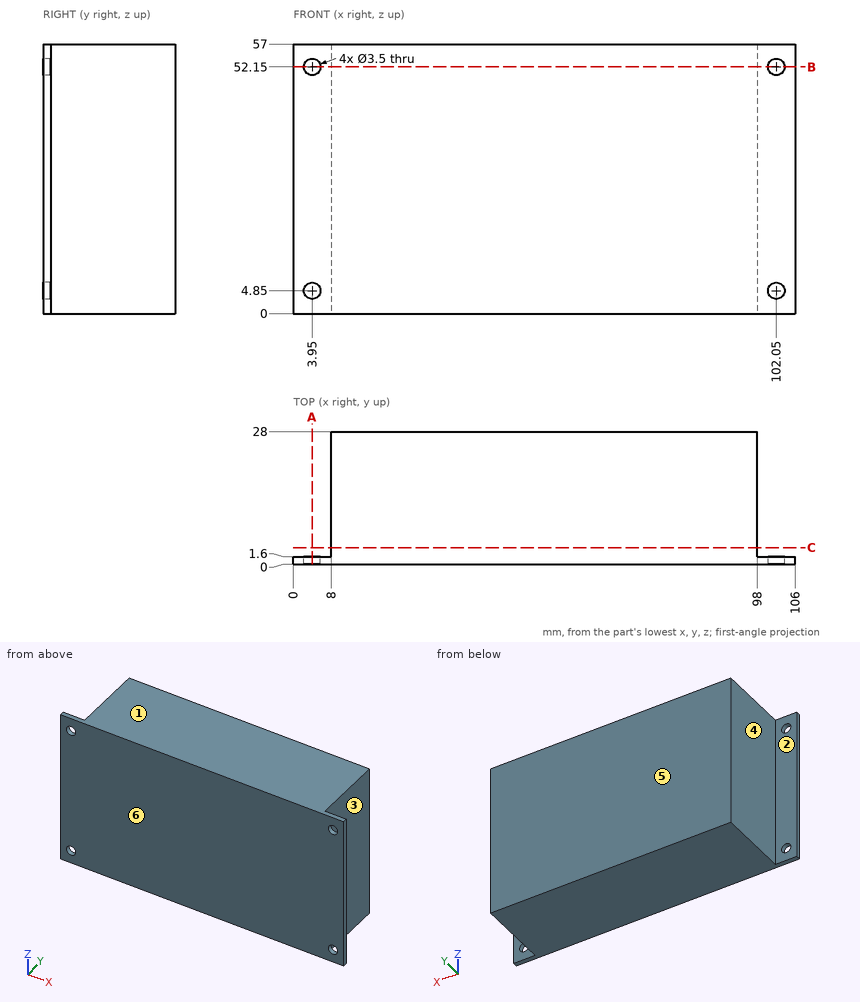
Source: three-view drawing plus pictorial views. Frame: mm from the lowest corner of the part. A direction names the side the tool comes from. Give positions to 0.01 mm unless a question says otherwise; leave off trailing zeros. Loops run counter-clockwise (first coordinate to the right, second up) from the corner with the lowest first, then second, coordinate; pieces in that order, holes last. Notation, with made-up numbers: (-24, 65.5) -> (31, 65.5) arc R22 cw to (31, 71.5) -> close; hole circle Ø5 at (25.25, 83). An arc over 180 degrees is marked (long way). Use a Markdown table: item, result. Add a question column.
(1) First-contact query: pin 1 Ø12 at (y, z) = (22, 25.5) entering from +X; pin 2 Ø6 at (x, z) = (92.5, 29.5) entering from -Y; pin 3 Ø4.5 at (x, z) = (3.95, 4.85) entering from +Y; pin 4 Ø1.5 at (y, z) = (6.5, 19) entering from -X. Flat tips, straight axial feed; report the tip coordinate or a pass-through.
(2) Ray query, line 1 (X direction, y = 0.5, z = 52.15); line 2 (X direction, y = 26.75, z = 33). Return the intervals inside material, ascending.
(3) Access query for the marked faces 1, 2 and 3. Directions: +Z, -Z, +X, -X, +Y, -Y. A direction counts if a zero-diameter tool reaches every point of the face in a straight line with its end or side. Return the directions, or none.
(4) Section query B-B (z = 52.15). Output: boundary loops of the cut face in (x, y).
(5) Pull-direction query (Y, two-part tool) for the marked faces 4, 5 and 6; classes: +Y half, -Y half, draft (parallel to the pull), parting line (faces both ways), or undercut.
(6) Section query C-C (y = 3.5). Output: boundary loops of the cut face in (x, z), then the cut area to 3 significant figures.
(7) Section query A-A (x = 3.95). Output: boundary loops of the cut face in (y, z).
Checked values:
| question | item | result |
|---|---|---|
| 1 | pin 1 | x = 98 |
| 1 | pin 2 | y = 0 |
| 1 | pin 3 | y = 1.6 |
| 1 | pin 4 | x = 8 |
| 2 | line 1 | 0 to 2.2, 5.7 to 100.3, 103.8 to 106 |
| 2 | line 2 | 8 to 98 |
| 3 | face 1 | +Z, +X, -X, +Y, -Y |
| 3 | face 2 | +Z, -Z, -X, +Y |
| 3 | face 3 | +Z, -Z, +X, +Y |
| 4 | outline | (0, 0) -> (2.2, 0) -> (2.2, 1.6) -> (0, 1.6) -> close; (5.7, 0) -> (100.3, 0) -> (100.3, 1.6) -> (98, 1.6) -> (98, 28) -> (8, 28) -> (8, 1.6) -> (5.7, 1.6) -> close; (103.8, 0) -> (106, 0) -> (106, 1.6) -> (103.8, 1.6) -> close |
| 5 | face 4 | draft |
| 5 | face 5 | +Y half |
| 5 | face 6 | -Y half |
| 6 | outline | (8, 0) -> (98, 0) -> (98, 57) -> (8, 57) -> close |
| 6 | area | 5,130 mm^2 |
| 7 | outline | (0, 0) -> (1.6, 0) -> (1.6, 3.1) -> (0, 3.1) -> close; (0, 6.6) -> (1.6, 6.6) -> (1.6, 50.4) -> (0, 50.4) -> close; (0, 53.9) -> (1.6, 53.9) -> (1.6, 57) -> (0, 57) -> close |
